from build123d import *

# Parameters (mm, degrees)
F1_DEPTH       = 76.2
F3_D           = 38.1
F3_CBORE_D     = 50.8
F3_CBORE_DEPTH = 12.7
F5_D           = 38.1
F5_CBORE_D     = 50.8
F5_CBORE_DEPTH = 12.7


with BuildPart() as f1:
    # F0 (on Front) → F1 (new body)
    with BuildSketch(Plane.XZ):
        with BuildLine():
            Line((-58.056168, 15.794694), (-58.056168, -60.405306))
            Line((-58.056168, -60.405306), (119.743832, -60.405306))
            Line((119.743832, -60.405306), (119.743832, -31.830306))
            Line((119.743832, -31.830306), (24.493832, -31.830306))
            Line((24.493832, -31.830306), (24.493832, 15.794694))
            ThreePointArc((24.493832, 15.794694), (12.404664, 44.980527), (-16.781168, 57.069694))
            ThreePointArc((-16.781168, 57.069694), (-45.967001, 44.980527), (-58.056168, 15.794694))
        make_face()
    extrude(amount=F1_DEPTH)

    # F3 (through all)
    with Locations(Plane.XZ.offset(76.2)):
        with Locations((-16.781168, 15.794694)):
            CounterBoreHole(F3_D / 2, F3_CBORE_D / 2, F3_CBORE_DEPTH)

    # F5 (through all)
    with Locations(Plane.XY.offset(-31.830306)):
        with Locations((81.643832, -38.1)):
            CounterBoreHole(F5_D / 2, F5_CBORE_D / 2, F5_CBORE_DEPTH)


solid = f1.part
Work out the finished part from the listing and answer in its coordinate system (mm). A direction names the side the tool comes from. Round coordinates to 2 decimals unless told otherwise and drop trailing zeros. Write each loop counter-clockwise with the first axis right and the second up, starting at its lowest first coordinate (ties: lowest second). Pieces come first, ordered by that corner, then holes. Notation, with made-up numbers: (23, 41) -> (52, 41) arc R18 cw to (52, 57) -> close; hole circle Ø2 at (51, 11.5). An arc over 180 degrees is marked (long way). Answer as CSV lines item,"result". Start each with the question number.
(1) Find the intervals of material crossed by probe 1 along X at (y, z) = (-31, 15); probe 2 along Z at (x, y) = (82.5, -62.5); probe 3 along X at (y, z) = (-44.5, -16), in increasing order.
(2) A tool of negligible diameter and unlimited length cuts with its end or side. For faces 1 (the flat face through (85, -19, -44.53)), 2 (the flat face through (30, -38, -60.405)), 3 (the flat face through (52, -38, -31.83)), 4 (the flat face through (-13, -63.5, 35)), from which of +Z, -Z, +X, -X, +Y, -Y can it reach the whole face along a straight path? Write none if from no direction.
(3) The part is cut by section B-B, the plane z = -52. Give the vertices of the cut face in (x, y).
(4) Each of these flat-tipped pins is pushed along its axis until it touches: pin 1 (8 mm diameter, centred on x = 92, y = -19.5, fed in from +Z); pin 2 (10 mm diameter, centred on x = 47.5, y = -47, fed in from +Z); pin 3 (24 mm diameter, centred on y = -39.5, z = -4.5, fed in from +X). Where does it stop, or does it pass through?
(5) The part is cut by section A-A, the plane y = -38.1. Give the vertices of the cut face in (x, z) (3 decimals).
(6) The mould has two halves that part along Y. Classify faces 5 (the flat face through (10, -76.2, -14)), 6 (the cylindrical face through (105.87, -30.47, -38.09)), 7 (the flat face through (10, 0, -14)), 8 (the flat face through (24.494, -38, -8)): +Y half, -Y half, draft (parallel to the pull), parting line (faces both ways), or undercut.
(7) The part is cut by section C-C, the plane y = -15. Give the vertices of the cut face in (x, z) (3 decimals), then the cut area to 3 significant figures.
(8) The part is cut by section D-D, the plane z = 11. Give the vertices of the cut face in (x, y), then the cut area to 3 significant figures.
Output values:
1,probe 1,"x = -58.06 to -35.81, 2.25 to 24.49"
1,probe 2,"z = -60.41 to -44.53"
1,probe 3,"x = -58.06 to 24.49"
2,face 1,"+Z"
2,face 2,"-Z, +X, -X, +Y, -Y"
2,face 3,"+Z, +X, +Y, -Y"
2,face 4,"-Y"
3,outline,"(-58.06, -76.2) -> (119.74, -76.2) -> (119.74, 0) -> (-58.06, 0) -> close; hole circle Ø38.1 at (81.64, -38.1)"
4,pin 1,"stops at z = -44.53"
4,pin 2,"stops at z = -31.83"
4,pin 3,"stops at x = 24.49"
5,outline,"(-58.056, -60.405) -> (62.594, -60.405) -> (62.594, -44.53) -> (56.244, -44.53) -> (56.244, -31.83) -> (24.494, -31.83) -> (24.494, 15.795) arc R41.275 ccw to (-16.781, 57.07) arc R41.275 ccw to (-58.056, 15.795) -> close; (100.694, -60.405) -> (119.744, -60.405) -> (119.744, -31.83) -> (107.044, -31.83) -> (107.044, -44.53) -> (100.694, -44.53) -> close; hole circle Ø38.1 at (-16.781, 15.795)"
6,face 5,"-Y half"
6,face 6,"undercut"
6,face 7,"+Y half"
6,face 8,"draft"
7,outline,"(-58.056, -60.405) -> (119.744, -60.405) -> (119.744, -31.83) -> (92.206, -31.83) -> (92.206, -44.53) -> (71.082, -44.53) -> (71.082, -31.83) -> (24.494, -31.83) -> (24.494, 15.795) arc R41.275 ccw to (-16.781, 57.07) arc R41.275 ccw to (-58.056, 15.795) -> close; hole circle Ø38.1 at (-16.781, 15.795)"
7,area,"10,300 mm²"
8,outline,"(-58.06, -76.2) -> (-41.72, -76.2) -> (-41.72, -63.5) -> (-35.22, -63.5) -> (-35.22, 0) -> (-58.06, 0) -> close; (1.66, -63.5) -> (8.16, -63.5) -> (8.16, -76.2) -> (24.49, -76.2) -> (24.49, 0) -> (1.66, 0) -> close"
8,area,"3,320 mm²"
